Verification items for the finished model (mm, model axes). A direction names the side the tool comes from. Round coordinates to 2 decimals unless told otherwise and drop trailing zeros. Write each loop counter-clockwise with the first axis right and the second up, starting at its lowest first coordinate (ties: lowest second). Pieces come first, ordered by that corner, then holes. Notation, with made-up numbers: M 36,9.25 L 79,9.25 A25 ccw 79,35.25 Z; hole C 61,39 d6. An arc over 180 degrees is marked long. One line per item, written item: value. Start each with the question number.
from build123d import *

# Parameters (mm, degrees)
PAD_DEPTH    = 115
POCKET_DEPTH = 15.322068
SKETCH002_W  = 15
SKETCH002_H  = 5
PAD001_DEPTH = 2
FILLET_R     = 3
FILLET001_R  = 2
CHAMFER_SIZE = 1
FILLET002_R  = 1
FILLET003_R  = 1
FILLET004_R  = 1
FILLET005_R  = 1


with BuildPart() as part:
    # Sketch → Pad (new body)
    with BuildSketch(Plane.XY):
        Polygon((-17.625, 0), (17.625, 0), (17.625, 2.25), (14.089466, 5.785534), (17.625, 9.321068), (17.625, 11.321068), (21.625, 11.321068), (21.625, -4), (-21.625, -4), (-21.625, 11.321068), (-17.625, 11.321068), (-17.625, 9.321068), (-14.089466, 5.785534), (-17.625, 2.25), align=None)
    extrude(amount=PAD_DEPTH)

    # Sketch001 (on Face8 of Pad) → Pocket (cut, through all)
    with BuildSketch(Plane.XZ.offset(4)):
        Polygon((7.5, 130), (7.5, 20), (48.935, 20), (48.935, 139.08), (-48.935, 139.08), (-48.935, 20), (-7.5, 20), (-7.5, 130), align=None)
    extrude(amount=-POCKET_DEPTH, mode=Mode.SUBTRACT)

    # Sketch002 (on Face1 of Pocket) → Pad001 (join)
    with BuildSketch(Plane(origin=(0, 0, 0), x_dir=(-1, 0, 0), z_dir=(0, 1, 0))):
        with Locations((0, 112.5)):
            Rectangle(SKETCH002_W, SKETCH002_H)
    extrude(amount=PAD001_DEPTH)

    # Fillet
    fillet_edges = [part.edges().sort_by_distance(p)[0] for p in [
        (21.625, 3.660534, 20),
        (21.625, 3.660534, 0),
        (-21.625, 3.660534, 0),
        (-21.625, 3.660534, 20),
        (-7.5, -2, 20),
        (7.5, -2, 20),
    ]]
    fillet(fillet_edges, radius=FILLET_R)

    # Fillet001
    fillet001_edges = [part.edges().sort_by_distance(p)[0] for p in [
        (-7.5, -2, 115),
        (7.5, -2, 115),
    ]]
    fillet(fillet001_edges, radius=FILLET001_R)

    # Chamfer
    chamfer_edges = [part.edges().sort_by_distance(p)[0] for p in [
        (7.5, -4, 68),
        (6.914214, -4, 114.414214),
        (8.37868, -4, 20.87868),
        (0, -4, 115),
        (14.5625, -4, 20),
        (-6.914214, -4, 114.414214),
        (20.74632, -4, 19.12132),
        (-7.5, -4, 68),
        (21.625, -4, 10),
        (-8.37868, -4, 20.87868),
        (20.74632, -4, 0.87868),
        (-14.5625, -4, 20),
        (0, -4, 0),
        (-20.74632, -4, 19.12132),
        (-20.74632, -4, 0.87868),
        (-21.625, -4, 10),
    ]]
    chamfer(chamfer_edges, length=CHAMFER_SIZE)

    # Fillet002
    fillet002_edges = [part.edges().sort_by_distance(p)[0] for p in [
        (0, 2, 115),
    ]]
    fillet(fillet002_edges, radius=FILLET002_R)

    # Fillet003
    fillet003_edges = [part.edges().sort_by_distance(p)[0] for p in [
        (-18.125, 11.321068, 0),
        (-20.74632, 11.321068, 0.87868),
        (-17.625, 11.321068, 10),
        (-21.625, 11.321068, 10),
        (-18.125, 11.321068, 20),
        (-20.74632, 11.321068, 19.12132),
        (18.125, 11.321068, 0),
        (20.74632, 11.321068, 0.87868),
        (17.625, 11.321068, 10),
        (21.625, 11.321068, 10),
        (18.125, 11.321068, 20),
        (20.74632, 11.321068, 19.12132),
    ]]
    fillet(fillet003_edges, radius=FILLET003_R)

    # Fillet004
    fillet004_edges = [part.edges().sort_by_distance(p)[0] for p in [
        (-7.5, 0, 66.5),
    ]]
    fillet(fillet004_edges, radius=FILLET004_R)

    # Fillet005
    fillet005_edges = [part.edges().sort_by_distance(p)[0] for p in [
        (7.5, 0, 66.5),
    ]]
    fillet(fillet005_edges, radius=FILLET005_R)


solid = part.part
1) Cross-section at A-A (y = 4.25). Record the boundary of the cut face in (x, z) (3 decimals), then the cut area to 3 significant figures.
2) Gauge pin test, flat ends, axial feed: pin 1 Ø9 at (x, y) = (14.5, 3) entering from +Z; pin 2 Ø10.5 at (x, z) = (1, 34) entering from +Y; pin 3 Ø1.5 at (x, y) = (15, 9.5) entering from +Z; pin 4 Ø2 at (y, z) = (-1, 51) entering from +X. Record the tip position at first contact, or that the pin passes through.
3) Cross-section at D-D (x = -2.5). Record the boundary of the cut face in (y, z), then the cut area to 3 significant figures.
4) Access from +Z, -Z, +X, -X, +Y, -Y to the whole of each face (thin tool, end or side, straight path). Record for faces 4 (the flat face through (-15.832, 4.043, 9.86)), 5 (the flat face through (-15.882, 7.578, 9.86)), 6 (the flat face through (7.5, -2, 67)).
5) Cross-section at B-B (x = 15.5). Record the boundary of the cut face in (y, z) (3 decimals), then the cut area to 3 significant figures.
6) Mould release check, pull along X, two halves, no side actions. Record for faces 1 (the conical face through (6.466, -3.618, 113.988)), 2 (the flat face through (0.1, -0.3, 0)), 3 (the flat face through (17.625, 1, 10)): pulls with the +X half, pulls with the -X half, needs draft (parallel to the pull), parting line crosses it, or undercut.
7) Cross-section at C-C (z = 40). Record the boundary of the cut face in (x, y).
8) Thickness scan on line 1 (Y direction, x = 2.5, z = 18.5); line 2 (Z direction, x = 18, y = 10); line 3 (X direction, y = -3, z = 41). Record the ranges inside material, lowest first.
Results below:
1. outline: M -21.625,3 A3 ccw -18.625,0 L -15.625,0 L -15.625,20 L -18.625,20 A3 ccw -21.625,17 Z; M 15.625,0 L 18.625,0 A3 ccw 21.625,3 L 21.625,17 A3 ccw 18.625,20 L 15.625,20 Z
1. area: 232 mm²
2. pin 1: stops at z = 20
2. pin 2: stops at y = 0
2. pin 3: passes through
2. pin 4: stops at x = 7.5
3. outline: M -4,1 L -3,0 L 0,0 L 0,110 L 2,110 L 2,114 A1 ccw 1,115 L -3,115 L -4,114 Z
3. area: 469 mm²
4. face 4: +Z, -Z
4. face 5: +Z, -Z, +Y
4. face 6: +Z, +X, +Y, -Y
5. outline: M -4,1 L -3,0 L 0,0 L 0,19 A1 ccw -1,20 L -3,20 L -4,19 Z; M 4.375,0 L 7.196,0 L 7.196,20 L 4.375,20 Z
5. area: 135 mm²
6. face 1: pulls with the +X half
6. face 2: needs draft
6. face 3: undercut
7. outline: M -7.5,-3 L -6.5,-4 L 6.5,-4 L 7.5,-3 L 7.5,-1 A1 ccw 6.5,0 L -6.5,0 A1 ccw -7.5,-1 Z
8. line 1: y = -4 to 0
8. line 2: z = 0 to 20
8. line 3: x = -7.5 to 7.5
